```python
from build123d import *

# Parameters (mm, degrees)
SKETCH1_R           = 8
BOSS_EXTRUDE1_DEPTH = 9
SKETCH3_W           = 60
SKETCH3_H           = 116
BOSS_EXTRUDE2_DEPTH = 30
SKETCH4_R           = 30
BOSS_EXTRUDE3_DEPTH = 60
SKETCH6_R           = 8
SKETCH6_R_2         = 4
BOSS_EXTRUDE4_DEPTH = 20
SKETCH7_W           = 53.624772313
SKETCH7_H           = 116
CUT_EXTRUDE2_DEPTH  = 189.729965909
SKETCH8_R           = 12
CUT_EXTRUDE3_DEPTH  = 189.729965909
BOSS_EXTRUDE5_START = -25
BOSS_EXTRUDE5_DEPTH = 25
SKETCH10_R          = 20
CUT_EXTRUDE4_DEPTH  = 20
SKETCH11_R          = 15
CUT_EXTRUDE5_DEPTH  = 20
SKETCH12_R          = 9
CUT_EXTRUDE6_DEPTH  = 181.828648262
SKETCH13_R          = 4
CUT_EXTRUDE7_DEPTH  = 31
CUT_EXTRUDE8_DEPTH  = 42


with BuildPart() as part:
    # Sketch1 → Boss-Extrude1 (new body)
    with BuildSketch(Plane(origin=(0, 0, 0), x_dir=(1, 0, 0), z_dir=(0, 1, 0))):
        with BuildLine():
            Line((40, -27), (40, 27))
            ThreePointArc((40, 27), (49.192388155, 49.192388155), (27, 40))
            Line((27, 40), (-27, 40))
            ThreePointArc((-27, 40), (-49.192388155, 49.192388155), (-40, 27))
            Line((-40, 27), (-40, -27))
            ThreePointArc((-40, -27), (-49.192388155, -49.192388155), (-27, -40))
            Line((-27, -40), (27, -40))
            ThreePointArc((27, -40), (49.192388155, -49.192388155), (40, -27))
        make_face()
        with Locations(Location((-40, 40, 0), (0, 0, 270))):
            Circle(SKETCH1_R, mode=Mode.SUBTRACT)
        with Locations(Location((-40, -40, 0), (0, 0, 270))):
            Circle(SKETCH1_R, mode=Mode.SUBTRACT)
        with Locations(Location((40, -40, 0), (0, 0, 270))):
            Circle(SKETCH1_R, mode=Mode.SUBTRACT)
        with Locations(Location((40, 40, 0), (0, 0, 270))):
            Circle(SKETCH1_R, mode=Mode.SUBTRACT)
    extrude(amount=BOSS_EXTRUDE1_DEPTH)

    # Sketch3 → Boss-Extrude2 (add, symmetric)
    with BuildSketch(Plane(origin=(0, 0, 0), x_dir=(0, 0, -1), z_dir=(1, 0, 0))):
        with Locations((0, 67)):
            Rectangle(SKETCH3_W, SKETCH3_H)
    extrude(amount=BOSS_EXTRUDE2_DEPTH, both=True)

    # Sketch4 → Boss-Extrude3 (add)
    with BuildSketch(Plane.XY.offset(30)):
        with Locations((0, 125)):
            Circle(SKETCH4_R)
    extrude(amount=-BOSS_EXTRUDE3_DEPTH)

    # Sketch6 → Boss-Extrude4 (add)
    with BuildSketch(Plane(origin=(0, 161, 0), x_dir=(1, 0, 0), z_dir=(0, 1, 0))):
        with Locations(Location((0, 0, 0), (0, 0, 270))):
            Circle(SKETCH6_R)
        with Locations(Location((0, 0, 0), (0, 0, 270))):
            Circle(SKETCH6_R_2, mode=Mode.SUBTRACT)
    extrude(amount=-BOSS_EXTRUDE4_DEPTH)

    # Sketch7 → Cut-Extrude2 (cut, through all)
    with BuildSketch(Plane.XY.offset(30)):
        with Locations((26.812386157, 103)):
            Rectangle(SKETCH7_W, SKETCH7_H)
    extrude(amount=-CUT_EXTRUDE2_DEPTH, mode=Mode.SUBTRACT)

    # Sketch8 → Cut-Extrude3 (cut, through all)
    with BuildSketch(Plane.XY.offset(30)):
        with Locations((0, 45)):
            Circle(SKETCH8_R)
    extrude(amount=-CUT_EXTRUDE3_DEPTH, mode=Mode.SUBTRACT)

    # Sketch9 → Boss-Extrude5 (add)
    with BuildSketch(Plane(origin=(0, 0, -15), x_dir=(-1, 0, 0), z_dir=(0, 0, -1)).offset(BOSS_EXTRUDE5_START)):
        with BuildLine():
            Line((-12, 45), (-7, 45))
            ThreePointArc((-7, 45), (4.949747468, 40.050252532), (0, 52))
            Line((0, 52), (0, 57))
            ThreePointArc((0, 57), (8.485281374, 36.514718626), (-12, 45))
        make_face()
    extrude(amount=BOSS_EXTRUDE5_DEPTH)

    # Sketch10 → Cut-Extrude4 (cut)
    with BuildSketch(Plane.XY.offset(30)):
        with Locations((0, 125)):
            Circle(SKETCH10_R)
    extrude(amount=-CUT_EXTRUDE4_DEPTH, mode=Mode.SUBTRACT)

    # Sketch11 → Cut-Extrude5 (cut)
    with BuildSketch(Plane.XY.offset(10)):
        with Locations((0, 125)):
            Circle(SKETCH11_R)
    extrude(amount=-CUT_EXTRUDE5_DEPTH, mode=Mode.SUBTRACT)

    # Sketch12 → Cut-Extrude6 (cut, through all)
    with BuildSketch(Plane.XY.offset(-10)):
        with Locations((0, 125)):
            Circle(SKETCH12_R)
    extrude(amount=-CUT_EXTRUDE6_DEPTH, mode=Mode.SUBTRACT)

    # Sketch13 → Cut-Extrude7 (cut)
    with BuildSketch(Plane(origin=(0, 161, 0), x_dir=(1, 0, 0), z_dir=(0, 1, 0))):
        Circle(SKETCH13_R)
    extrude(amount=-CUT_EXTRUDE7_DEPTH, mode=Mode.SUBTRACT)

    # Sketch14 → Cut-Extrude8 (cut)
    with BuildSketch(Plane.XY.offset(21)):
        with BuildLine():
            Line((19, 45), (30, 45))
            Line((30, 45), (30, 9))
            Line((30, 9), (0, 9))
            Line((0, 9), (0, 26))
            ThreePointArc((0, 26), (13.435028843, 31.564971157), (19, 45))
        make_face()
    extrude(amount=-CUT_EXTRUDE8_DEPTH, mode=Mode.SUBTRACT)


solid = part.part
```
Read the model definition and answer for the solid it produces. Units are mm, in the model's axes. A direction names the side the tool comes from. Round coordinates to 2 decimals unless told otherwise and drop trailing zeros. Write each loop counter-clockwise with the first axis right and the second up, starting at its lowest first coordinate (ties: lowest second). Pieces come first, ordered by that corner, then holes. Notation, with made-up numbers: (9.25, -23) -> (31.25, -23) arc R29 cw to (31.25, 7) -> close; hole circle Ø9 at (37.25, 6.5). An arc over 180 degrees is marked (long way). Answer in a Markdown table with one row per item. Add a question column.
1) Which of the six approach directions +Z, -Z, +X, -X, +Y, -Y give full straight-line access (tool end or side, diameter ignored) to faces 5 (the face through (0, 4, -40)), 6 (the face through (-7, 67, 30)), 7 (the face through (30, 27, -25)), 8 (the face through (-8.76, 36.8, -22.39))?
2) Find section C-C, the plane x = 14. Determine the outline of the cut face in (y, z).
3) Consider line 1 (Z direction, x = 14.5, y = 18.5); line 2 (Y direction, x = -5.5, z = 6); line 3 (X direction, y = 13, z = -21.5). Determine where each line is inside the solid, lowest interval first.
4) Find section A-A, the plane x = -44.5. Determine the outline of the cut face in (y, z).
5) Given P1, Ø6, axis at y = 94, z = 26, coming from the +X side; P2, Ø11.5, axis at x = 16, z = -12.5, coming from the +Y side; P3, Ø1.5, axis at y = 87, z = 19, coming from the -X side; P4, Ø18, axis at x = 12.5, y = 116.5, coming from the +Z side, each flat-ended and moving along its own axis, determine where each tip first touches the part or whether it passes through.
6) Find section D-D, the plane y = 14. Determine the outline of the cut face in (x, z), and give its area (3 significant figures).
7) Find section B-B, the plane z = -44. Determine the outline of the cut face in (x, y), and give its area (3 significant figures).
8) Determine the mould class of faces 1 (the face through (-40, 4, 0)), 2 (the face through (-15, 125, 0)), 3 (the face through (-1, 0, -1)), 4 (the face through (16, 45, 0)) for opening direction Y: pulls with the +Y half, pulls with the -Y half, needs draft (parallel to the pull), parting line crosses it, or undercut.
Findings below:
| question | item | result |
|---|---|---|
| 1 | face 5 | -Z, +Y, -Y |
| 1 | face 6 | +Z, +X, -X, +Y |
| 1 | face 7 | +Z, -Z, +X, +Y |
| 1 | face 8 | -Z |
| 2 | outline | (0, -40) -> (9, -40) -> (9, -30) -> (45, -30) -> (45, 30) -> (9, 30) -> (9, 40) -> (0, 40) -> close; hole (9, -21) -> (32.15, -21) -> (32.15, 21) -> (9, 21) -> close |
| 3 | line 1 | -30 to -21, 21 to 30 |
| 3 | line 2 | 0 to 40.67, 49.33 to 111.04, 138.96 to 154.49 |
| 3 | line 3 | -30 to 30 |
| 4 | outline | (0, -52.2) -> (9, -52.2) -> (9, -46.61) -> (0, -46.61) -> close; (0, -33.39) -> (9, -33.39) -> (9, -27.8) -> (0, -27.8) -> close; (0, 27.8) -> (9, 27.8) -> (9, 33.39) -> (0, 33.39) -> close; (0, 46.61) -> (9, 46.61) -> (9, 52.2) -> (0, 52.2) -> close |
| 5 | P1 | x = 0 |
| 5 | P2 | y = 45 |
| 5 | P3 | x = -30 |
| 5 | P4 | through |
| 6 | outline | (-30, -30) -> (30, -30) -> (30, -21) -> (0, -21) -> (0, 21) -> (30, 21) -> (30, 30) -> (-30, 30) -> close |
| 6 | area | 2,340 mm² |
| 7 | outline | (-52.37, 0) -> (-46.93, 0) -> (-46.93, 9) -> (-52.37, 9) -> close; (-33.07, 0) -> (-27.63, 0) -> (-27.63, 9) -> (-33.07, 9) -> close; (27.63, 0) -> (33.07, 0) -> (33.07, 9) -> (27.63, 9) -> close; (46.93, 0) -> (52.37, 0) -> (52.37, 9) -> (46.93, 9) -> close |
| 7 | area | 196 mm² |
| 8 | face 1 | needs draft |
| 8 | face 2 | undercut |
| 8 | face 3 | pulls with the -Y half |
| 8 | face 4 | pulls with the +Y half |
